Geometry: final body of the model. Coordinates: model frame, mm. Face numbers are marked on the shaded views. A direction names the side the tool comes from. Give positions to 0.01 mm unless a question says otherwise; leave off trailing zeros. Loops run counter-clockwise (first coordinate to the right, second up) from the corner with the lowest first, then second, coordinate; pieces in that order, holes last.
from build123d import *
from build123d.topology import SkipClean

# Parameters (mm, degrees)
ESQUISSE1_R                  = 23.35
BOSS_EXTRU_1_DEPTH           = 5
ESQUISSE9_R                  = 1.5
ESQUISSE9_R_2                = 2
ESQUISSE9_R_3                = 2.25
ESQUISSE9_W                  = 35
ESQUISSE9_H                  = 15
ENL_V_MAT_EXTRU_2_DEPTH      = 5
ESQUISSE9_3_W                = 25
ESQUISSE9_3_H                = 2
BOSS_EXTRU_2_DEPTH           = 15
BOSS_EXTRU_3_DEPTH           = 2
BOSS_EXTRU_4_DEPTH           = 3.1
BOSS_EXTRU_5_DEPTH           = 2
BOSS_EXTRU_6_DEPTH           = 12
ESQUISSE15_R                 = 23.35
ESQUISSE15_R_2               = 21.35
BOSS_EXTRU_7_DEPTH           = 2.5
ENL_V_MAT_EXTRU_4_DEPTH      = 39.606281872
ENL_V_MAT_EXTRU_4_DEPTH_BACK = 4
ESQUISSE16_W                 = 7
ESQUISSE16_H                 = 5


with BuildPart() as part:
    # Esquisse1 → Boss.-Extru.1 (new body)
    with BuildSketch(Plane(origin=(0, 0, 0), x_dir=(1, 0, 0), z_dir=(0, 1, 0))):
        with Locations(Location((0, 0, 0), (0, 0, 270))):
            Circle(ESQUISSE1_R)
    extrude(amount=BOSS_EXTRU_1_DEPTH)

    # Esquisse9 → Enl_v. mat.-Extru.2 (cut)
    with BuildSketch(Plane(origin=(0, 5, 0), x_dir=(1, 0, 0), z_dir=(0, 1, 0))):
        with Locations(Location((-13.185409426, 13.185409426, 0), (0, 0, 270))):
            Circle(ESQUISSE9_R)
        with Locations(Location((13.185409426, 13.185409426, 0), (0, 0, 270))):
            Circle(ESQUISSE9_R)
        with Locations(Location((13.185409426, -13.185409426, 0), (0, 0, 270))):
            Circle(ESQUISSE9_R)
        with Locations(Location((-13.185409426, -13.185409426, 0), (0, 0, 270))):
            Circle(ESQUISSE9_R)
        with Locations(Location((0, 15.303635433, 0), (0, 0, 270))):
            Circle(ESQUISSE9_R_2)
        with Locations(Location((-7, 15.303635433, 0), (0, 0, 270))):
            Circle(ESQUISSE9_R_3)
        Rectangle(ESQUISSE9_W, ESQUISSE9_H)
    extrude(amount=-ENL_V_MAT_EXTRU_2_DEPTH, mode=Mode.SUBTRACT)

    # Esquisse9_3 → Boss.-Extru.2 (add)
    with BuildSketch(Plane(origin=(0, 5, 0), x_dir=(1, 0, 0), z_dir=(0, 1, 0))):
        with Locations((0, 8.5)):
            Rectangle(ESQUISSE9_3_W, ESQUISSE9_3_H)
        with Locations((0, -8.5)):
            Rectangle(ESQUISSE9_3_W, ESQUISSE9_3_H)
    extrude(amount=BOSS_EXTRU_2_DEPTH)

    # Esquisse11 → Boss.-Extru.3 (add)
    with BuildSketch(Plane(origin=(0, 20, 0), x_dir=(1, 0, 0), z_dir=(0, 1, 0))):
        Polygon((-12.5, 9.5), (-12.5, -9.5), (-12.5, -12.5), (12.5, -12.5), (12.5, 12.5), (-12.5, 12.5), align=None)
    extrude(amount=-BOSS_EXTRU_3_DEPTH)

    # Esquisse12 → Boss.-Extru.4 (add)
    with BuildSketch(Plane(origin=(0, 20, 0), x_dir=(1, 0, 0), z_dir=(0, 1, 0))):
        Polygon((-12.5, -12.5), (-10, -12.5), (-10, 10), (10, 10), (10, -12.5), (12.5, -12.5), (12.5, 12.5), (-12.5, 12.5), align=None)
    extrude(amount=BOSS_EXTRU_4_DEPTH)

    # Esquisse13 → Boss.-Extru.5 (add)
    with BuildSketch(Plane(origin=(0, 23.1, 0), x_dir=(1, 0, 0), z_dir=(0, 1, 0))):
        Polygon((-9, -12.5), (-9, 6.5), (9, 6.5), (9, -12.5), (12.5, -12.5), (12.5, 12.5), (-12.5, 12.5), (-12.5, -12.5), align=None)
    extrude(amount=BOSS_EXTRU_5_DEPTH)

    # Esquisse14 → Boss.-Extru.6 (add)
    with BuildSketch(Plane(origin=(0, 5, 0), x_dir=(1, 0, 0), z_dir=(0, 1, 0))):
        with BuildLine():
            Line((10, -18.863257937), (10, -21.100296206))
            ThreePointArc((10, -21.100296206), (16.510943341, -16.510943341), (21.100296206, -10))
            Line((21.100296206, -10), (18.863257937, -10))
            ThreePointArc((18.863257937, -10), (15.096729778, -15.096729778), (10, -18.863257937))
        make_face()
        with BuildLine():
            Line((-18.863257937, -10), (-21.100296206, -10))
            ThreePointArc((-21.100296206, -10), (-16.510943341, -16.510943341), (-10, -21.100296206))
            Line((-10, -21.100296206), (-10, -18.863257937))
            ThreePointArc((-10, -18.863257937), (-15.096729778, -15.096729778), (-18.863257937, -10))
        make_face()
        with BuildLine():
            ThreePointArc((-10, 21.100296206), (-16.510943341, 16.510943341), (-21.100296206, 10))
            Line((-21.100296206, 10), (-18.863257937, 10))
            ThreePointArc((-18.863257937, 10), (-15.096729778, 15.096729778), (-10, 18.863257937))
            Line((-10, 18.863257937), (-10, 21.100296206))
        make_face()
        with BuildLine():
            ThreePointArc((21.100296206, 10), (16.510943341, 16.510943341), (10, 21.100296206))
            Line((10, 21.100296206), (10, 18.863257937))
            ThreePointArc((10, 18.863257937), (15.096729778, 15.096729778), (18.863257937, 10))
            Line((18.863257937, 10), (21.100296206, 10))
        make_face()
    extrude(amount=BOSS_EXTRU_6_DEPTH)

    # Esquisse15 → Boss.-Extru.7 (add)
    with SkipClean():  # the faces are left unmerged after this step: merging them gives an invalid solid
        with BuildSketch(Plane(origin=(0, 17, 0), x_dir=(1, 0, 0), z_dir=(0, 1, 0))):
            with Locations(Location((0, 0, 0), (0, 0, 270))):
                Circle(ESQUISSE15_R)
            with Locations(Location((0, 0, 0), (0, 0, 62.070545626))):
                Circle(ESQUISSE15_R_2, mode=Mode.SUBTRACT)
        extrude(amount=BOSS_EXTRU_7_DEPTH)

    # Esquisse16 → Enl_v. mat.-Extru.4 (cut, two sides: drawn at the far end of the back side and taken through both)
    with SkipClean():  # the faces are left unmerged after this step: merging them gives an invalid solid
        with BuildSketch(Plane(origin=(0, 20, 0), x_dir=(1, 0, 0), z_dir=(0, 1, 0)).offset(-ENL_V_MAT_EXTRU_4_DEPTH_BACK)):
            with Locations((0, -10)):
                Rectangle(ESQUISSE16_W, ESQUISSE16_H)
        extrude(amount=ENL_V_MAT_EXTRU_4_DEPTH + ENL_V_MAT_EXTRU_4_DEPTH_BACK, mode=Mode.SUBTRACT)


solid = part.part
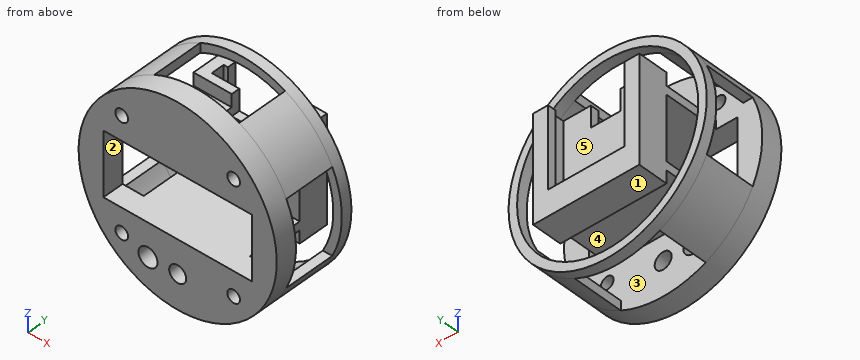
Item 1: Section query C-C on y = 2.5. Return loops of the section in (x, z), plus the area to 3 significant figures.
Values follow:
outline: circle Ø46.7 at (0, 0); hole (-17.5, -7.5) - (17.5, -7.5) - (17.5, 7.5) - (-17.5, 7.5) - close; hole circle Ø3 at (-13.19, -13.19); hole circle Ø3 at (-13.19, 13.19); hole circle Ø4.5 at (-7, -15.3); hole circle Ø4 at (0, -15.3); hole circle Ø3 at (13.19, -13.19); hole circle Ø3 at (13.19, 13.19)
area: 1,130 mm2
Item 2: Section query A-A on x = 0. Give the number of separate pieces and of enclosed holes in the cut face, plus the area to 3 significant figures.
Values follow:
separate pieces: 5
enclosed holes: 0
area: 256 mm2
Item 3: Section query B-B on z = 0. Return loops of the section in (x, y).
Values follow:
outline: (-23.35, 0) - (-17.5, 0) - (-17.5, 5) - (-23.35, 5) - close; (-23.35, 17) - (-21.35, 17) - (-21.35, 19.5) - (-23.35, 19.5) - close; (-12.5, 18) - (12.5, 18) - (12.5, 25.1) - (9, 25.1) - (9, 23.1) - (10, 23.1) - (10, 20) - (-10, 20) - (-10, 23.1) - (-9, 23.1) - (-9, 25.1) - (-12.5, 25.1) - close; (17.5, 0) - (23.35, 0) - (23.35, 5) - (17.5, 5) - close; (21.35, 17) - (23.35, 17) - (23.35, 19.5) - (21.35, 19.5) - close
Item 4: Set-up query: the marked faces 1, 2 and 3. Return all of +Z, -Z, +X, -X, +Y, -Y with unobstructed straight access to the full face (end or side cutting, diameter ignored); none if empty.
Values follow:
face 1: +Y
face 2: +Y, -Y
face 3: none
Item 5: Pin query (flat end, axial travel): pin 1 (0.6 mm diameter, centred on y = 24, z = 1, fed in from -X); pin 2 (14.5 mm diameter, centred on x = 4.5, y = 10.5, fed in from +Z); pin 3 (1.1 mm diameter, centred on x = -19.5, y = 13, fed in from +Z); pin 4 (6 mm diameter, centred on x = -7.5, y = 13, fed in from +Z). Return the tip coordinate at first contact, or that it passes through.
Values follow:
pin 1: stops at x = -12.5
pin 2: stops at z = 23.35
pin 3: stops at z = 13.64
pin 4: stops at z = 21.1
Item 6: Section query D-D on x = 14. Return loops of the section in (y, z), plus the area to 3 significant figures.
Values follow:
outline: (0, -18.69) - (19.5, -18.69) - (19.5, -16.12) - (5, -16.12) - (5, -14.44) - (0, -14.44) - close; (0, -11.93) - (5, -11.93) - (5, -7.5) - (0, -7.5) - close; (0, 7.5) - (5, 7.5) - (5, 11.93) - (0, 11.93) - close; (0, 14.44) - (5, 14.44) - (5, 16.12) - (19.5, 16.12) - (19.5, 18.69) - (0, 18.69) - close
area: 161 mm2
Item 7: Draft query along Z for the marked faces 4 and 5. Return one class per face: +Z half, -Z half, draft (parallel to the pull), parting line (faces both ways), or undercut.
Values follow:
face 4: undercut
face 5: draft
Item 8: Ray query, probe 1 along Z at (x, y) = (0, 18.8); probe 2 along Y at (x, z) = (7, -11.5); probe 3 along Z at (x, y) = (-6, 4). Return the intervals inside material, ascending.
Values follow:
probe 1: z = -23.35 to -21.35, -12.5 to 7.5, 21.35 to 23.35
probe 2: y = 0 to 5, 18 to 25.1
probe 3: z = -22.57 to -17.32, -13.29 to -7.5, 7.5 to 22.57
